Input: part model. Units: mm. Frame: model coordinates. A direction names the side the tool comes from. Round coordinates to 2 decimals unless told otherwise and drop trailing zeros. Loops run counter-clockwise (first coordinate to the right, second up) from the corner with the lowest first, then second, coordinate; pieces in that order, holes last.
(1) Access query for faces 4 (the face through (-9.4, 36, -12)), 5 (the face through (-10.4, 36, -23)), 6 (the face through (11, 2, -3)). Directions: +Z, -Z, +X, -X, +Y, -Y. A direction counts if a zero-diameter tool reaches every point of the face in a straight line with its end or side. Return the directions, or none.
(2) Line query: line 1 (X direction, y = 0.75, z = -12.25); line 2 (X direction, y = 16.5, z = -23.5); line 3 (Y direction, x = -12, z = 11). Output: solid intervals per line, ascending.
(3) Cut plane D-D, the plane x = -2. Output: boundary loops of the cut face in (y, z), and give its area (3 significant figures).
(4) Draft query along Z for faces 1 (the face through (19, 36, -29.35)), 2 (the face through (9.4, 36, 3)), 3 (the face through (10.49, 0.986, 9.213)). Return one class per face: released by +Z, released by -Z, zero draft, split by the parting line, or undercut.
(5) Cut plane C-C, the plane y = 21.5. Output: boundary loops of the cut face in (x, z).
(6) Cut plane B-B, the plane z = 8.45. Output: boundary loops of the cut face in (x, y), and give its area (3 significant figures).
(7) First-contact query: pin 1 Ø2 at (y, z) = (21.5, -2) entering from +X; pin 2 Ø2.5 at (x, y) = (17, 36) entering from -Z; pin 3 Ø2.5 at (x, z) = (-21, -17) entering from -Y. Flat tips, straight axial feed; report the tip coordinate or a pass-through.
(8) Cut plane A-A, the plane z = -1. Output: boundary loops of the cut face in (x, y), and give its area (3 significant figures).
from build123d import *

# Parameters (mm, degrees)
SKETCH1_R               = 0.8
BOSS_EXTRUDE2_DEPTH     = 2
BOSS_EXTRUDE4_DEPTH     = 35.2
BOSS_EXTRUDE7_OUTLINE_R = 0.8
BOSS_EXTRUDE7_DEPTH     = 37.2
SKETCH1_10_R            = 0.8
CUT_EXTRUDE6_DEPTH      = 34.2
SKETCH1_11_R            = 0.8
BOSS_EXTRUDE8_DEPTH     = 2
SKETCH2_W               = 9
SKETCH2_H               = 8
SKETCH2_H_2             = 10
BOSS_EXTRUDE9_DEPTH     = 3
CHAMFER1_SIZE           = 10


# Read off the part's stored shape, not the designer's step: Boss-Extrude7
with BuildPart() as part:
    # Sketch1 → Boss-Extrude2 (new body)
    with BuildSketch(Plane(origin=(0, 0, 0), x_dir=(1, 0, 0), z_dir=(0, 1, 0))):
        Polygon((-10.4, 16.242178951), (-10.4, 30.95), (-14.6, 30.95), (-14.6, -16.65), (14.6, -16.65), (14.6, 30.95), (10.4, 30.95), (10.4, 16.242178951), (7.2, 13.042178951), (7.2, -14.85), (-7.2, -14.85), (-7.2, 13.042178951), align=None)
        with Locations(Location((-10.25, -8.45, 0), (0, 0, 270))):
            Circle(SKETCH1_R, mode=Mode.SUBTRACT)
        with Locations(Location((-10.25, 12.25, 0), (0, 0, 270))):
            Circle(SKETCH1_R, mode=Mode.SUBTRACT)
        with Locations(Location((-10.25, -12.25, 0), (0, 0, 270))):
            Circle(SKETCH1_R, mode=Mode.SUBTRACT)
        with Locations(Location((10.25, -8.45, 0), (0, 0, 270))):
            Circle(SKETCH1_R, mode=Mode.SUBTRACT)
        with Locations(Location((10.25, -12.25, 0), (0, 0, 270))):
            Circle(SKETCH1_R, mode=Mode.SUBTRACT)
        with Locations(Location((10.25, 12.25, 0), (0, 0, 270))):
            Circle(SKETCH1_R, mode=Mode.SUBTRACT)
    extrude(amount=BOSS_EXTRUDE2_DEPTH)

    # Sketch1<6> → Boss-Extrude4 (add)
    with BuildSketch(Plane(origin=(0, 0, 0), x_dir=(1, 0, 0), z_dir=(0, 1, 0))):
        Polygon((-12.8, -14.85), (-12.8, 30.95), (-14.6, 30.95), (-14.6, -16.65), (14.6, -16.65), (14.6, 30.95), (12.8, 30.95), (12.8, -14.85), align=None)
    extrude(amount=BOSS_EXTRUDE4_DEPTH)

    # Boss-Extrude7 outline → Boss-Extrude7 (add)
    with BuildSketch(Plane(origin=(0, 0, 0), x_dir=(1, 0, 0), z_dir=(0, 1, 0))):
        Polygon((14.6, -16.65), (14.6, 30.95), (10.4, 30.95), (10.4, 16.242178951), (9.4, 15.242178951), (9.4, 9.2), (10.3, 9.2), (10.3, 3.8), (9.4, 3.8), (9.4, -9.55), (-9.4, -9.55), (-9.4, 3.9), (-10.3, 3.9), (-10.3, 9.2), (-9.4, 9.2), (-9.4, 15.242178951), (-10.4, 16.242178951), (-10.4, 30.95), (-14.6, 30.95), (-14.6, -16.65), align=None)
        with Locations((-10.25, -12.25)):
            Circle(BOSS_EXTRUDE7_OUTLINE_R, mode=Mode.SUBTRACT)
        with Locations((10.25, -12.25)):
            Circle(BOSS_EXTRUDE7_OUTLINE_R, mode=Mode.SUBTRACT)
    extrude(amount=BOSS_EXTRUDE7_DEPTH)

    # Sketch1<10> → Cut-Extrude6 (cut)
    with BuildSketch(Plane(origin=(0, 0, 0), x_dir=(1, 0, 0), z_dir=(0, 1, 0))):
        Polygon((-10.4, 16.242178951), (-10.4, 30.95), (-12.8, 30.95), (-12.8, -14.85), (12.8, -14.85), (12.8, 30.95), (10.4, 30.95), (10.4, 16.242178951), (7.2, 13.042178951), (7.2, -9.55), (-7.2, -9.55), (-7.2, 13.042178951), align=None)
        with Locations(Location((-10.25, -12.25, 0), (0, 0, 270))):
            Circle(SKETCH1_10_R, mode=Mode.SUBTRACT)
        with Locations(Location((10.25, -12.25, 0), (0, 0, 270))):
            Circle(SKETCH1_10_R, mode=Mode.SUBTRACT)
    extrude(amount=CUT_EXTRUDE6_DEPTH, mode=Mode.SUBTRACT)

    # Sketch1<11> → Boss-Extrude8 (add)
    # profile 1 of 2: a face of its own
    with BuildSketch(Plane(origin=(0, 0, 0), x_dir=(1, 0, 0), z_dir=(0, 1, 0))):
        Polygon((-10.4, 16.242178951), (-10.4, 30.95), (-12.8, 30.95), (-12.8, -14.85), (-7.2, -14.85), (-7.2, 13.042178951), align=None)
        with Locations(Location((-10.25, -8.45, 0), (0, 0, 270))):
            Circle(SKETCH1_11_R, mode=Mode.SUBTRACT)
        with Locations(Location((-10.25, 12.25, 0), (0, 0, 270))):
            Circle(SKETCH1_11_R, mode=Mode.SUBTRACT)
    # profile 2 of 2: a face of its own
    with BuildSketch(Plane(origin=(0, 0, 0), x_dir=(1, 0, 0), z_dir=(0, 1, 0))):
        Polygon((7.2, -14.85), (12.8, -14.85), (12.8, 30.95), (10.4, 30.95), (10.4, 16.242178951), (7.2, 13.042178951), align=None)
        with Locations(Location((10.25, -8.45, 0), (0, 0, 270))):
            Circle(SKETCH1_11_R, mode=Mode.SUBTRACT)
        with Locations(Location((10.25, 12.25, 0), (0, 0, 270))):
            Circle(SKETCH1_11_R, mode=Mode.SUBTRACT)
    extrude(amount=BOSS_EXTRUDE8_DEPTH)

    # Sketch2 → Boss-Extrude9 (add)
    # profile 1 of 4: a face of its own
    with BuildSketch(Plane(origin=(0, 37.2, 0), x_dir=(1, 0, 0), z_dir=(0, 1, 0))):
        with Locations((-19.1, 25.35)):
            Rectangle(SKETCH2_W, SKETCH2_H)
        with BuildLine():
            ThreePointArc((-17.46862915, 24.48137085), (-18.6, 21.75), (-19.73137085, 24.48137085))
            Line((-19.73137085, 24.48137085), (-18.6, 25.6127417))
            Line((-18.6, 25.6127417), (-17.46862915, 24.48137085))
        make_face(mode=Mode.SUBTRACT)
    # profile 2 of 4: a face of its own
    with BuildSketch(Plane(origin=(0, 37.2, 0), x_dir=(1, 0, 0), z_dir=(0, 1, 0))):
        with Locations((19.1, 25.35)):
            Rectangle(SKETCH2_W, SKETCH2_H)
        with BuildLine():
            Line((18.6, 25.6127417), (19.73137085, 24.48137085))
            ThreePointArc((19.73137085, 24.48137085), (18.6, 21.75), (17.46862915, 24.48137085))
            Line((17.46862915, 24.48137085), (18.6, 25.6127417))
        make_face(mode=Mode.SUBTRACT)
    # profile 3 of 4: a face of its own
    with BuildSketch(Plane(origin=(0, 37.2, 0), x_dir=(1, 0, 0), z_dir=(0, 1, 0))):
        with Locations((-19.1, -11.65)):
            Rectangle(SKETCH2_W, SKETCH2_H_2)
        with BuildLine():
            Line((-19.73137085, -11.51862915), (-18.6, -10.3872583))
            Line((-18.6, -10.3872583), (-17.46862915, -11.51862915))
            ThreePointArc((-17.46862915, -11.51862915), (-18.6, -14.25), (-19.73137085, -11.51862915))
        make_face(mode=Mode.SUBTRACT)
    # profile 4 of 4: a face of its own
    with BuildSketch(Plane(origin=(0, 37.2, 0), x_dir=(1, 0, 0), z_dir=(0, 1, 0))):
        with Locations((19.1, -11.65)):
            Rectangle(SKETCH2_W, SKETCH2_H_2)
        with BuildLine():
            Line((17.46862915, -11.51862915), (18.6, -10.3872583))
            Line((18.6, -10.3872583), (19.73137085, -11.51862915))
            ThreePointArc((19.73137085, -11.51862915), (18.6, -14.25), (17.46862915, -11.51862915))
        make_face(mode=Mode.SUBTRACT)
    extrude(amount=-BOSS_EXTRUDE9_DEPTH)

    # Chamfer1
    # the kernel refuses this chamfer: 10 mm, written as the material it adds along each edge
    with BuildSketch(Plane(origin=(14.6, 37.2, -21.35), x_dir=(0.9996219169112968, 0, -0.027495876610586667), z_dir=(0, -1, 0))) as chamfer1_piece_1_section:
        Polygon((CHAMFER1_SIZE * 0.999621916911, CHAMFER1_SIZE * 0.0274958766106), (-CHAMFER1_SIZE * 0.0274958766106, CHAMFER1_SIZE * 0.999621916911), (0, 0), align=None)
    chamfer1_piece_1 = extrude(amount=3, mode=Mode.PRIVATE)
    chamfer1_piece_1 = split(chamfer1_piece_1, bisect_by=Plane(origin=(23.6, 35.7, -17.990992529), z_dir=(-1, 0, 0)), keep=Keep.TOP, mode=Mode.PRIVATE)
    add(chamfer1_piece_1)
    with BuildSketch(Plane(origin=(-14.6, 37.2, -21.35), x_dir=(-0.9996219169112968, 0, -0.027495876610586324), z_dir=(0, -1, 0))) as chamfer1_piece_2_section:
        Polygon((CHAMFER1_SIZE * 0.999621916911, -CHAMFER1_SIZE * 0.0274958766106), (-CHAMFER1_SIZE * 0.0274958766106, -CHAMFER1_SIZE * 0.999621916911), (0, 0), align=None)
    chamfer1_piece_2 = extrude(amount=3, mode=Mode.PRIVATE)
    chamfer1_piece_2 = split(chamfer1_piece_2, bisect_by=Plane(origin=(-23.6, 35.7, -17.990992529), z_dir=(1, 0, 0)), keep=Keep.TOP, mode=Mode.PRIVATE)
    add(chamfer1_piece_2)


solid = part.part
Reported:
1. face 4: -Z, +Y
1. face 5: -Z, +Y, -Y
1. face 6: -Z
2. line 1: x = -14.6 to -11.05, -9.45 to -7.2, 7.2 to 9.45, 11.05 to 14.6
2. line 2: x = -14.6 to -12.8, 12.8 to 14.6
2. line 3: y = 0 to 2, 34.2 to 37.2
3. outline: (0, 14.85) - (34.2, 14.85) - (34.2, 9.55) - (37.2, 9.55) - (37.2, 16.65) - (0, 16.65) - close
3. area: 82.9 mm2
4. face 1: released by -Z
4. face 2: zero draft
4. face 3: undercut
5. outline: (-14.6, -30.95) - (-12.8, -30.95) - (-12.8, 14.85) - (12.8, 14.85) - (12.8, -30.95) - (14.6, -30.95) - (14.6, 16.65) - (-14.6, 16.65) - close
6. outline: (-23.6, 34.2) - (-14.6, 34.2) - (-14.6, 0) - (-11.05, 0) - (-11.05, 2) - (-12.8, 2) - (-12.8, 34.2) - (-9.4, 34.2) - (-9.4, 37.2) - (-23.6, 37.2) - close; (-9.45, 0) - (-7.2, 0) - (-7.2, 2) - (-9.45, 2) - close; (7.2, 0) - (9.45, 0) - (9.45, 2) - (7.2, 2) - close; (9.4, 34.2) - (12.8, 34.2) - (12.8, 2) - (11.05, 2) - (11.05, 0) - (14.6, 0) - (14.6, 34.2) - (23.6, 34.2) - (23.6, 37.2) - (9.4, 37.2) - close
6. area: 224 mm2
7. pin 1: stops at x = 14.6
7. pin 2: stops at z = -29.35
7. pin 3: stops at y = 34.2
8. outline: (-14.6, 0) - (-7.2, 0) - (-7.2, 2) - (-12.8, 2) - (-12.8, 34.2) - (-9.4, 34.2) - (-9.4, 37.2) - (-14.6, 37.2) - close; (7.2, 0) - (14.6, 0) - (14.6, 37.2) - (9.4, 37.2) - (9.4, 34.2) - (12.8, 34.2) - (12.8, 2) - (7.2, 2) - close
8. area: 177 mm2
